```python
from build123d import *

# Parameters (mm, degrees)
SKETCH2_W           = 30
SKETCH2_H           = 16
BOSS_EXTRUDE1_DEPTH = 12
SKETCH3_R           = 2
CUT_EXTRUDE1_DEPTH  = 21.808652047
FILLET1_R           = 1.5
FILLET2_R           = 0.8


with BuildPart() as part:
    # Sketch2 → Boss-Extrude1 (new body)
    with BuildSketch(Plane(origin=(0, 0, 0), x_dir=(1, 0, 0), z_dir=(0, 1, 0))):
        Rectangle(SKETCH2_W, SKETCH2_H)
    extrude(amount=BOSS_EXTRUDE1_DEPTH)

    # Sketch3 → Cut-Extrude1 (cut, through all)
    with BuildSketch(Plane(origin=(0, 12, 0), x_dir=(1, 0, 0), z_dir=(0, 1, 0))):
        with Locations(Location((0, 0, 0), (0, 0, 270))):
            Circle(SKETCH3_R)
    extrude(amount=-CUT_EXTRUDE1_DEPTH, mode=Mode.SUBTRACT)

    # Fillet1
    fillet1_edges = [part.edges().sort_by_distance(p)[0] for p in [
        (15, 6, 8),
        (-15, 6, 8),
        (-15, 6, -8),
        (15, 6, -8),
    ]]
    fillet(fillet1_edges, radius=FILLET1_R)

    # Fillet2
    fillet2_edges = [part.edges().sort_by_distance(p)[0] for p in [
        (0, 12, 8),
        (-15, 12, 0),
        (15, 12, 0),
        (0, 12, -8),
        (14.560660172, 12, 7.560660172),
        (14.560660172, 12, -7.560660172),
        (-14.560660172, 12, -7.560660172),
        (-14.560660172, 12, 7.560660172),
    ]]
    fillet(fillet2_edges, radius=FILLET2_R)


solid = part.part
```
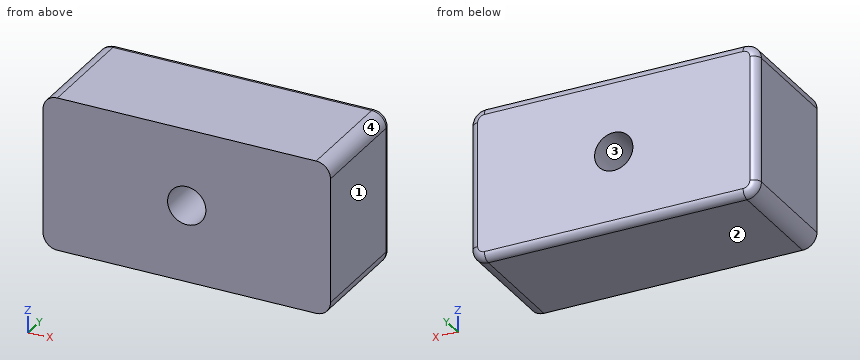
Part model, mm, in its own coordinate system. Face numbers are marked on the shaded views. Round coordinates to 2 decimals unless told otherwise and drop trailing zeros. Loops run counter-clockwise (first coordinate to the right, second up) from the corner with the lowest first, then second, coordinate; pieces in that order, holes last.
Item 1: Cut at C-C, the plane y = 9.5. Give the cut face in (x, z).
Item 2: Drill centre lines: line 1 (X direction, y = 3.75, z = 0); line 2 (Y direction, x = -12, z = 7.25); line 3 (X direction, y = 6.5, z = 0.5). Where is each one in solid material? Low to high.
Item 3: Mould opens along Z. For the marked faces 1, 2, 3 and 4 say: +Z half, -Z half, draft (parallel to the pull), parting line (faces both ways), or undercut.
Item 4: Drop a flat-ended pin along its axis: P1, Ø3, axis at x = 0, z = 0, coming from the -Y side. Give the stop position or say it passes through.
Item 5: Cut at A-A, the plane z = 0. Give the cut face in (x, y).
Item 6: Cut at B-B, the plane x = 0. Give the cut face in (y, z), then the cut area to 3 significant figures.
A:
1. outline: (-15, -6.5) arc R1.5 ccw to (-13.5, -8) - (13.5, -8) arc R1.5 ccw to (15, -6.5) - (15, 6.5) arc R1.5 ccw to (13.5, 8) - (-13.5, 8) arc R1.5 ccw to (-15, 6.5) - close; hole circle Ø4 at (0, 0)
2. line 1: x = -15 to -2, 2 to 15
2. line 2: y = 0 to 12
2. line 3: x = -15 to -1.94, 1.94 to 15
3. face 1: draft
3. face 2: -Z half
3. face 3: undercut
3. face 4: +Z half
4. P1: passes through
5. outline: (-15, 0) - (-2, 0) - (-2, 12) - (-14.2, 12) arc R0.8 ccw to (-15, 11.2) - close; (2, 0) - (15, 0) - (15, 11.2) arc R0.8 ccw to (14.2, 12) - (2, 12) - close
6. outline: (0, -8) - (11.2, -8) arc R0.8 ccw to (12, -7.2) - (12, -2) - (0, -2) - close; (0, 2) - (12, 2) - (12, 7.2) arc R0.8 ccw to (11.2, 8) - (0, 8) - close
6. area: 144 mm2
